The listing builds one solid part. Answer for the finished solid, in the listing's coordinates (mm). A direction names the side the tool comes from. Coordinates: 2 decimals unless noted, no trailing zeros. Write each loop counter-clockwise with the first axis right and the second up, starting at its lowest first coordinate (ties: lowest second). Pieces come first, ordered by that corner, then holes.
Autodesk Inventor part; units mm, degrees
ref_plane "YZ Plane" through (0, 0, 0) normal (1, 0, 0) x (0, 1, 0)
ref_plane "XZ Plane" through (0, 0, 0) normal (0, 1, 0) x (-1, 0, 0)
ref_plane "XY Plane" through (0, 0, 0) normal (0, 0, 1) x (1, 0, 0)
sketch "Sketch1" plane through (0, 0, 0) normal (0, 1, 0) x (-1, 0, 0)
  line L0 (-18.669, 18.669) -> (18.669, 18.669)
  line L1 (18.669, 18.669) -> (18.669, -18.669)
  line L2 (18.669, -18.669) -> (-18.669, -18.669)
  line L3 (-18.669, -18.669) -> (-18.669, 18.669)
  line L4 (-18.669, 18.669) -> (18.669, -18.669) construction
  line L5 (18.669, 18.669) -> (-18.669, -18.669) construction
  point P0 (0, 0)
  dimension "d0" = 37.338
extrude "Extrusion1" add sketch "Sketch1" along normal blind 14.224
sketch "Sketch2" plane through (18.669, 0, 18.669) normal (1, 0, 0) x (0, 0, -1)
  point P0 (18.669, 0)
sketch "Sketch3" plane through (0, 14.224, 0) normal (0, 1, 0) x (1, 0, 0)
  circle A0 centre (-17.526, -17.526) radius 1.143
  line L0 (-18.669, 18.669) -> (-18.669, -18.669)
  line L1 (-18.669, -18.669) -> (18.669, -18.669)
  circle A1 centre (-17.526, 17.526) radius 1.143
  circle A2 centre (17.526, 17.526) radius 1.143
  circle A3 centre (17.526, -17.526) radius 1.143
  line L2 (18.669, 18.669) -> (-18.669, 18.669)
  line L3 (18.669, -18.669) -> (18.669, 18.669)
  point P0 (0, 0)
  dimension "d3" = 2.286
  dimension "d4" = 2.286
  dimension "d5" = 2.286
  dimension "d6" = 2.286
extrude "Extrusion2" add sketch "Sketch3" along normal blind 3.556 contours A0 | A1 | A3 | A2
sketch "Sketch4" plane through (-17.526, 17.78, 17.526) normal (0, 1, 0) x (1, 0, 0)
  circle A0 centre (0, 0) radius 0.75
  circle A1 centre (35.052, 0) radius 0.75
  circle A2 centre (35.052, 35.052) radius 0.75
  circle A3 centre (0, 35.052) radius 0.75
  point P0 (17.526, 17.526)
  dimension "d9" = 1.5
  dimension "d10" = 1.5
  dimension "d11" = 1.5
  dimension "d12" = 1.5
extrude "Extrusion3" cut sketch "Sketch4" against normal blind 3.556
properties part number "Sensor_Release_Magnet"
Q1. Given pin 1 (0.8 mm diameter, centred on x = -17.5, z = 17.5, fed in from +Y); pin 2 (0.6 mm diameter, centred on x = -18, z = -18, fed in from +Y); pin 3 (2 mm diameter, centred on y = 16, z = -6, fed in from +X), each flat-ended and moving along its own axis, determine where each tip first touches the part or whether it passes through.
Answers below:
pin 1: stops at y = 14.22
pin 2: stops at y = 17.78
pin 3: passes through
Q2. Determine the mould class of faces 1 (the face through (-18.669, 7, 0)), 2 (the face through (-17.5, 14.224, -17.5)), 3 (the face through (0, 0, 0)) for opening direction X: released by +X, released by -X, zero draft, split by the parting line, or undercut.
Answers below:
face 1: released by -X
face 2: undercut
face 3: zero draft
Q3. Which of the six approach directions +Z, -Z, +X, -X, +Y, -Y give full straight-line access (tool end or side, diameter ignored) to faces 4 (the face through (-18.4, 14.224, 18.5)), 5 (the face through (18.5, 14.224, 18.4)), 6 (the face through (-18.5, 14.224, -18.4)), 7 (the face through (0, 7, 18.669)), 8 (the face through (16.384, 15.977, -17.476))?
Answers below:
face 4: +Z, -X, +Y
face 5: +Z, +X, +Y
face 6: -Z, -X, +Y
face 7: +Z, +X, -X, +Y, -Y
face 8: +Y
Q4. The part is cut by section A-A, the plane z = 10. Write down the section's boundary in (x, y).
Answers below:
outline: (-18.67, 0) - (18.67, 0) - (18.67, 14.22) - (-18.67, 14.22) - close
Q5. Find the intervals of material crossed by probe 1 along Y at (x, z) = (-10, 9), in increasing order.
Answers below:
probe 1: y = 0 to 14.22
Q6. The part is cut by section B-B, the plane x = -7.5. Write down the section's boundary in (y, z).
Answers below:
outline: (0, -18.67) - (14.22, -18.67) - (14.22, 18.67) - (0, 18.67) - close
